from build123d import *

# Parameters (mm, degrees)
SKETCH1_W           = 45
SKETCH1_H           = 6
BOSS_EXTRUDE1_DEPTH = 20
SKETCH2_W           = 6
SKETCH2_H           = 45
BOSS_EXTRUDE2_DEPTH = 26
SKETCH3_R           = 2.65
CUT_EXTRUDE1_DEPTH  = 26
SKETCH4_R           = 2.65
CUT_EXTRUDE2_DEPTH  = 26
FILLET1_R           = 5
SKETCH5_W           = 6
SKETCH5_H           = 26
BOSS_EXTRUDE3_DEPTH = 20
SKETCH8_R           = 2.15
BOSS_EXTRUDE6_DEPTH = 0.4
BOSS_EXTRUDE5_START = 0.4
SKETCH7_R           = 2.15
BOSS_EXTRUDE5_DEPTH = 0.4
SKETCH6_R           = 1.5
CUT_EXTRUDE3_DEPTH  = 47.885498824
FILLET2_R           = 20
FILLET3_R           = 6
FILLET4_R           = 0.3
FILLET5_R           = 0.3
CUT_EXTRUDE4_DEPTH  = 4.5


with BuildPart() as part:
    # Sketch1 → Boss-Extrude1 (new body)
    with BuildSketch(Plane(origin=(0, 0, 0), x_dir=(0, 0, -1), z_dir=(1, 0, 0))):
        with Locations((22.5, 3)):
            Rectangle(SKETCH1_W, SKETCH1_H)
    extrude(amount=-BOSS_EXTRUDE1_DEPTH)

    # Sketch2 → Boss-Extrude2 (add)
    with BuildSketch(Plane(origin=(0, 6, 0), x_dir=(1, 0, 0), z_dir=(0, 1, 0))):
        with Locations((3, 22.5)):
            Rectangle(SKETCH2_W, SKETCH2_H)
    extrude(amount=-BOSS_EXTRUDE2_DEPTH)

    # Sketch3 → Cut-Extrude1 (cut)
    with BuildSketch(Plane(origin=(0, 6, 0), x_dir=(1, 0, 0), z_dir=(0, 1, 0))):
        with Locations(Location((-10, 7, 0), (0, 0, 270))):
            Circle(SKETCH3_R)
        with Locations(Location((-10, 38, 0), (0, 0, 270))):
            Circle(SKETCH3_R)
    extrude(amount=-CUT_EXTRUDE1_DEPTH, mode=Mode.SUBTRACT)

    # Sketch4 → Cut-Extrude2 (cut)
    with BuildSketch(Plane(origin=(6, 0, 0), x_dir=(0, 0, -1), z_dir=(1, 0, 0))):
        with Locations((7, -10)):
            Circle(SKETCH4_R)
        with Locations((38, -10)):
            Circle(SKETCH4_R)
    extrude(amount=-CUT_EXTRUDE2_DEPTH, mode=Mode.SUBTRACT)

    # Fillet1
    fillet1_edges = [part.edges().sort_by_distance(p)[0] for p in [
        (-20, 3, -45),
        (3, -20, -45),
        (3, -20, 0),
        (-20, 3, 0),
    ]]
    fillet(fillet1_edges, radius=FILLET1_R)

    # Sketch5 → Boss-Extrude3 (add)
    with BuildSketch(Plane(origin=(6, 0, 0), x_dir=(0, 0, -1), z_dir=(1, 0, 0))):
        with Locations((30.5, -7)):
            Rectangle(SKETCH5_W, SKETCH5_H)
        with Locations((14.5, -7)):
            Rectangle(SKETCH5_W, SKETCH5_H)
    extrude(amount=BOSS_EXTRUDE3_DEPTH)

    # Sketch8 → Boss-Extrude6 (add)
    with BuildSketch(Plane.XY.offset(-27.5)):
        with Locations(Location((16, -4, 0), (0, 0, 90))):
            Circle(SKETCH8_R)
    extrude(amount=BOSS_EXTRUDE6_DEPTH)

    # Sketch7 → Boss-Extrude5 (add)
    with BuildSketch(Plane(origin=(0, 0, -17.5), x_dir=(-1, 0, 0), z_dir=(0, 0, -1)).offset(BOSS_EXTRUDE5_START)):
        with Locations(Location((-16, -4, 0), (0, 0, 90))):
            Circle(SKETCH7_R)
    extrude(amount=-BOSS_EXTRUDE5_DEPTH)

    # Sketch6 → Cut-Extrude3 (cut, through all)
    with BuildSketch(Plane.XY.offset(-11.5)):
        with Locations((16, -4)):
            Circle(SKETCH6_R)
    extrude(amount=-CUT_EXTRUDE3_DEPTH, mode=Mode.SUBTRACT)

    # Fillet2
    fillet2_edges = [part.edges().sort_by_distance(p)[0] for p in [
        (26, -20, -14.5),
        (26, -20, -30.5),
    ]]
    fillet(fillet2_edges, radius=FILLET2_R)

    # Fillet3
    fillet3_edges = [part.edges().sort_by_distance(p)[0] for p in [
        (26, 6, -14.5),
        (26, 6, -30.5),
    ]]
    fillet(fillet3_edges, radius=FILLET3_R - 0.0001)  # a hair under: the kernel refuses the full size

    # Fillet4
    fillet4_edges = [part.edges().sort_by_distance(p)[0] for p in [
        (16, -6.15, -27.1),
    ]]
    fillet(fillet4_edges, radius=FILLET4_R)

    # Fillet5
    fillet5_edges = [part.edges().sort_by_distance(p)[0] for p in [
        (16, -6.15, -17.9),
    ]]
    fillet(fillet5_edges, radius=FILLET5_R)

    # Sketch9 → Cut-Extrude4 (cut)
    with BuildSketch(Plane.XY.offset(-11.5)):
        Polygon((14.267949192, -1), (12.535898385, -4), (14.267949192, -7), (17.732050808, -7), (19.464101615, -4), (17.732050808, -1), align=None)
    extrude(amount=-CUT_EXTRUDE4_DEPTH, mode=Mode.SUBTRACT)


solid = part.part
Geometry check sheet. Reference: the model listing, model coordinates, mm. A direction names the side the tool comes from. Coordinates: 2 decimals unless noted, no trailing zeros. Order: outer loops, then holes, each group sorted by start corner. A loop starts at its lowest first (then second) coordinate and runs counter-clockwise, first axis right, second up. Notation, with made-up numbers: (-40, -24) - (0, -24) arc R20 cw to (0, 3) - close; hole circle Ø5 at (41.5, 40). An arc over 180 degrees is marked (long way). Answer in a Markdown table with one row per item. Add a question column.
1) Cross-section at C-C, the plane y = -10. Record the cut outline in (x, z).
2) Cross-section at D-D, the plane x = 16. State how many separate pieces and enclosed holes the cut face has, then the cut area to 3 significant figures.
3) Cross-section at B-B, the plane z = -7. Record the cut outline in (x, y).
4) Material ranges on line 1 along Z through (x, y) = (15, -12.75); line 2 along Y through (x, z) = (3.45, -7); line 3 along Z through (x, y) = (0.5, -11.5), recorded low to high. Write a range as [from, to].
5) Release check for a two-part mould opening along Z. For faces 3 (the flat face through (6, -7, -22)), 4 (the flat face through (6, -7, -39)), 5 (the cylindrical face through (3, -18, -1)) record: +Z half, -Z half, draft (parallel to the pull), parting line (faces both ways), or undercut.
6) Gauge pin test, flat ends, axial feed: P1, Ø8.5, axis at y = -10, z = -7, coming from the -X side; P2, Ø10, axis at x = 21, y = -0.5, coming from the +Z side; P3, Ø4, axis at x = 16, y = -4, coming from the -Z side; P4, Ø1.1, axis at x = 15.5, y = -4.5, coming from the +Z side. Record the tip position at first contact, or that the pin passes through.
7) Cross-section at A-A, the plane x = -10. Record the cut outline in (y, z).
8) Set-up check for faces 1 (the cylindrical face through (-11.612, 3.042, -9.103)), 2 (the flat face through (16, -1, -14)): record each of +Z, -Z, +X, -X, +Y, -Y from which the full face is reachable in a straight line by a thin tool's end or side.
Check result:
| question | item | result |
|---|---|---|
| 1 | outline | (0, -45) - (6, -45) - (6, -40.65) - (0, -40.65) - close; (0, -35.35) - (6, -35.35) - (6, -33.5) - (23.32, -33.5) - (23.32, -27.5) - (6, -27.5) - (6, -17.5) - (23.32, -17.5) - (23.32, -11.5) - (6, -11.5) - (6, -9.65) - (0, -9.65) - close; (0, -4.35) - (6, -4.35) - (6, 0) - (0, 0) - close |
| 2 | separate pieces | 4 |
| 2 | enclosed holes | 0 |
| 2 | area | 231 mm² |
| 3 | outline | (-20, 0) - (-12.65, 0) - (-12.65, 6) - (-20, 6) - close; (-7.35, 0) - (0, 0) - (0, -7.35) - (6, -7.35) - (6, 6) - (-7.35, 6) - close; (0, -20) - (6, -20) - (6, -12.65) - (0, -12.65) - close |
| 4 | line 1 | z = [-33.5, -27.5], [-17.5, -11.5] |
| 4 | line 2 | y = [-20, -12.65], [-7.35, 6] |
| 4 | line 3 | z = [-45, -40.18], [-35.82, -9.18], [-4.82, 0] |
| 5 | face 3 | undercut |
| 5 | face 4 | draft |
| 5 | face 5 | +Z half |
| 6 | P1 | stops at x = 0 |
| 6 | P2 | stops at z = -11.5 |
| 6 | P3 | stops at z = -33.5 |
| 6 | P4 | passes through |
| 7 | outline | (0, -45) - (6, -45) - (6, -40.65) - (0, -40.65) - close; (0, -35.35) - (6, -35.35) - (6, -9.65) - (0, -9.65) - close; (0, -4.35) - (6, -4.35) - (6, 0) - (0, 0) - close |
| 8 | face 1 | +Y, -Y |
| 8 | face 2 | +Z |
